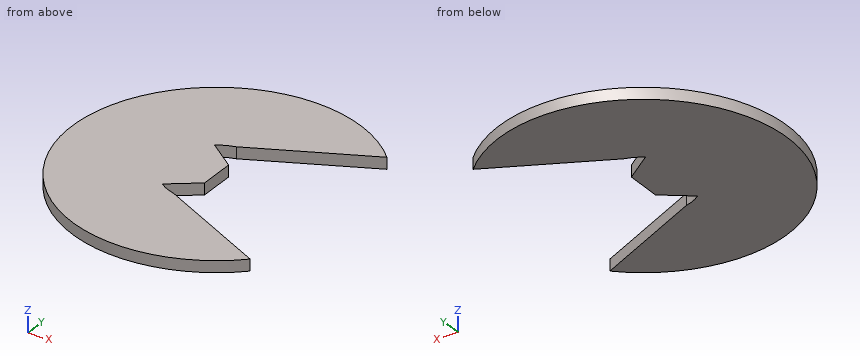
```python
from build123d import *

# Parameters (mm, degrees)
SKETCH1_R           = 3.75
BOSS_EXTRUDE1_DEPTH = 0.3
CUT_EXTRUDE2_DEPTH  = 1.3


with BuildPart() as part:
    # Sketch1 → Boss-Extrude1 (new body)
    with BuildSketch(Plane.XY):
        Circle(SKETCH1_R)
    extrude(amount=BOSS_EXTRUDE1_DEPTH)

    # Sketch2 → Cut-Extrude2 (cut, through all)
    with BuildSketch(Plane.XY.offset(0.3)):
        with BuildLine():
            Line((0, 0.466411964), (-0.73212486, 1.013160002))
            ThreePointArc((-0.73212486, 1.013160002), (-0.526515635, 1.133702468), (-0.301764614, 1.21302849))
            Line((-0.301764614, 1.21302849), (2.653016072, 2.650284083))
            ThreePointArc((2.653016072, 2.650284083), (3.75, 0), (2.653016072, -2.650284083))
            Line((2.653016072, -2.650284083), (-0.301764614, -1.21302849))
            ThreePointArc((-0.301764614, -1.21302849), (-0.526515635, -1.133702468), (-0.73212486, -1.013160002))
            Line((-0.73212486, -1.013160002), (0, -0.466411964))
            Line((0, -0.466411964), (0, 0.466411964))
        make_face()
    extrude(amount=-CUT_EXTRUDE2_DEPTH, mode=Mode.SUBTRACT)


solid = part.part
```
The listing builds one solid part. Answer for the finished solid, in the listing's coordinates (mm). Give positions to 0.01 mm unless a question says otherwise; leave off trailing zeros. Order: outer loops, then holes, each group sorted by start corner. A loop starts at its lowest first (then second) coordinate and runs counter-clockwise, first axis right, second up. Notation, with made-up numbers: (20, 12) -> (55, 12) arc R21 cw to (55, 22) -> close; hole circle Ø7 at (30.5, -2.75). An arc over 180 degrees is marked (long way). Answer as a JSON object with one key per item and string values. Group by question number.
Item 1: The part is cut by section A-A on x = 0.75. Write down the section's boundary in (y, z), and give its area (3 significant figures).
Item 2: The part is cut by section D-D on x = -1.75. Write down the section's boundary in (y, z).
Item 3: Consider L1, parallel to Y at x = -0.5, z = 0.2; L2, parallel to Y at x = 1, z = 0.2; L3, parallel to Y at x = -3.25, z = 0.2. Determine where each line is inside the solid, lowest interval first. Write a range as from..to.
Item 4: The part is cut by section C-C on y = 0. Write down the section's boundary in (x, z).
Item 5: The part is cut by section B-B on z = 0.05. Write down the section's boundary in (x, y).
Item 6: A flat-ended cylindrical pin translates along its axis: pin 1 (3 mm diameter, centred on x = -2, y = -1, fed in from -Z). Find the tip coordinate at first contact, or state that the pin passes through.
Result set:
{
 "1": {"outline": "(-3.67, 0) -> (-1.72, 0) -> (-1.72, 0.3) -> (-3.67, 0.3) -> close; (1.72, 0) -> (3.67, 0) -> (3.67, 0.3) -> (1.72, 0.3) -> close", "area": "1.17 mm²"},
 "2": {"outline": "(-3.32, 0) -> (3.32, 0) -> (3.32, 0.3) -> (-3.32, 0.3) -> close"},
 "3": {"L1": "-3.72..-1.15, -0.84..0.84, 1.15..3.72", "L2": "-3.61..-1.85, 1.85..3.61", "L3": "-1.87..1.87"},
 "4": {"outline": "(-3.75, 0) -> (0, 0) -> (0, 0.3) -> (-3.75, 0.3) -> close"},
 "5": {"outline": "(-0.73, -1.01) -> (0, -0.47) -> (0, 0.47) -> (-0.73, 1.01) arc R1.25 cw to (-0.3, 1.21) -> (2.65, 2.65) arc R3.75 ccw (long way) to (2.65, -2.65) -> (-0.3, -1.21) arc R1.25 cw to start"},
 "6": {"pin 1": "z = 0"}
}
